Here's how the part is built. I have some questions about the finished solid (model axes, mm). Coordinates: 2 decimals unless noted, no trailing zeros. Loops run counter-clockwise (first coordinate to the right, second up) from the corner with the lowest first, then second, coordinate; pieces in that order, holes last.
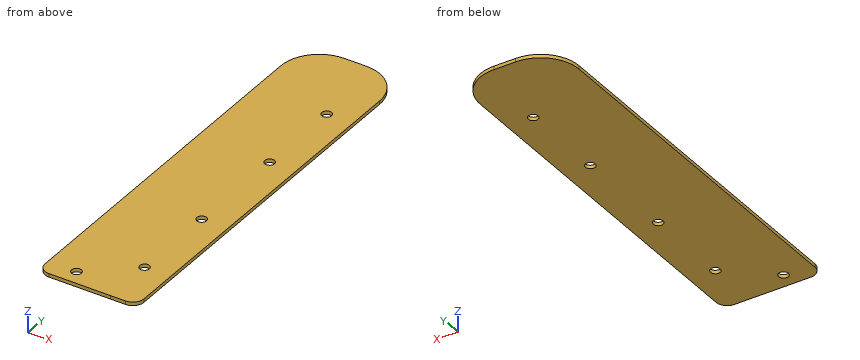
from build123d import *

# Parameters (mm, degrees)
SKETCH1_R           = 2.2479
BOSS_EXTRUDE2_DEPTH = 1.6002


with BuildPart() as part:
    # Sketch1 → Boss-Extrude2 (new body)
    with BuildSketch(Plane.XY):
        with BuildLine():
            Line((45.72, 5.08), (45.72, 172.72))
            ThreePointArc((45.72, 172.72), (40.512358569, 185.292358569), (27.94, 190.5))
            Line((27.94, 190.5), (17.78, 190.5))
            ThreePointArc((17.78, 190.5), (5.207641431, 185.292358569), (0, 172.72))
            Line((0, 172.72), (0, 5.08))
            ThreePointArc((0, 5.08), (1.503493452, 1.526611814), (5.070014314, 0.054542149))
            Line((5.070014314, 0.054542149), (33.655, 0))
            Line((33.655, 0), (40.64, 0))
            ThreePointArc((40.64, 0), (44.232102448, 1.487897552), (45.72, 5.08))
        make_face()
        with Locations((33.655, 24.13)):
            Circle(SKETCH1_R, mode=Mode.SUBTRACT)
        with Locations((33.655, 64.77)):
            Circle(SKETCH1_R, mode=Mode.SUBTRACT)
        with Locations((33.655, 113.03)):
            Circle(SKETCH1_R, mode=Mode.SUBTRACT)
        with Locations((33.655, 153.67)):
            Circle(SKETCH1_R, mode=Mode.SUBTRACT)
        with Locations((13.208, 7.15102725)):
            Circle(SKETCH1_R, mode=Mode.SUBTRACT)
    extrude(amount=BOSS_EXTRUDE2_DEPTH)


solid = part.part
Q1. Will this pin go through, and if not, where does the flat tip stop? P1, Ø3.5, axis at x = 33.655, y = 113.03, coming from the +Z side.
Q2. Please list where these lines run through material, in increasing order: probe 1 along Y at (x, z) = (32, 0.95); probe 2 along Y at (x, z) = (34, 0.8); probe 3 along Y at (x, z) = (30, 0.95).
Q3. Suppose I cut it at B-B on z = 1. Write out the boundary of the cut face in (x, y) (3 decimals).
Q4. Suppose I cut it at A-A on y = 113.03. Write out the boundary of the cut face in (x, z), and give its area (3 significant figures).
Check values:
1. P1: passes through
2. probe 1: y = 0 to 22.61, 25.65 to 63.25, 66.29 to 111.51, 114.55 to 152.15, 155.19 to 190.03
2. probe 2: y = 0 to 21.91, 26.35 to 62.55, 66.99 to 110.81, 115.25 to 151.45, 155.89 to 189.44
2. probe 3: y = 0.01 to 190.38
3. outline: (0, 5.08) arc R5.08 ccw to (5.07, 0.055) - (33.655, 0) - (40.64, 0) arc R5.08 ccw to (45.72, 5.08) - (45.72, 172.72) arc R17.78 ccw to (27.94, 190.5) - (17.78, 190.5) arc R17.78 ccw to (0, 172.72) - close; hole circle Ø4.496 at (13.208, 7.151); hole circle Ø4.496 at (33.655, 24.13); hole circle Ø4.496 at (33.655, 64.77); hole circle Ø4.496 at (33.655, 113.03); hole circle Ø4.496 at (33.655, 153.67)
4. outline: (0, 0) - (31.41, 0) - (31.41, 1.6) - (0, 1.6) - close; (35.9, 0) - (45.72, 0) - (45.72, 1.6) - (35.9, 1.6) - close
4. area: 66.0 mm2
